Autodesk Inventor part; units mm, degrees
ref_plane "YZ Plane" through (0, 0, 0) normal (1, 0, 0) x (0, 1, 0)
ref_plane "XZ Plane" through (0, 0, 0) normal (0, 1, 0) x (-1, 0, 0)
ref_plane "XY Plane" through (0, 0, 0) normal (0, 0, 1) x (1, 0, 0)
sketch "Sketch1" plane through (0, 0, 0) normal (0, 0, 1) x (1, 0, 0)
  circle A0 centre (-0.2626, 0.8226) radius 5.775
  line L0 (-5.743, 8.5976) -> (11.2384, 8.5976)
  arc A1 (8.5691, -6.944) -> (11.2384, 8.5976) centre (11.2384, 0.5976) ccw
  line L1 (8.5691, -6.944) -> (-5.9413, -0.2275)
  line L2 (-5.743, 6.5976) -> (11.2384, 6.5976)
  arc A2 (9.3184, -5.0869) -> (11.2384, 6.5976) centre (11.2384, 0.5976) ccw
  line L3 (9.3184, -5.0869) -> (-5.9413, 1.9763)
  line L4 (-5.743, 8.5976) -> (-5.743, 6.5976)
  line L5 (-5.9413, 1.9763) -> (-5.9413, -0.2275)
  point P0 (0, 0)
  dimension "d6" = 11.55
  dimension "d0" = 6
  dimension "d2" = 2
  dimension "d3" = 90
extrude "Extrusion1" add sketch "Sketch1" along normal blind 10 contours L2 L4 L0 A1 L1 A0 L3 A2 | A0 L1 L5 L3 | A0 L5 L3
properties part number "01_Laser_Clamp_OnOffSwitch"
Could you check a few things on this model? Use its own coordinates, in mm. A direction names the side the tool comes from. Give positions to 0.01 mm unless a question says otherwise; leave off trailing zeros. Write each loop counter-clockwise with the first axis right and the second up, starting at its lowest first coordinate (ties: lowest second). Pieces come first, ordered by that corner, then holes. Notation, with made-up numbers: (76.25, 63.25) - (124.25, 63.25) arc R36 cw to (124.25, 100.25) - close; hole circle Ø3 at (3.25, -2). An arc over 180 degrees is marked (long way). Use CSV: the item, a comma, the result in double quotes. Start each with the question number.
Item 1: For faces 4 (the face through (6, -4, 10)), 5 (the face through (-5.743, 8, 5)), 6 (the face through (1.795, -1.605, 4.93)), 7 (the face through (1.415, -3.633, 4.93)), 8 (the face through (3, 6.598, 5)), which set-ups out of +Z, -Z, +X, -X, +Y, -Y let a thin tool reach every point of the face, with its end or its side?
Item 2: I'm going to push flat-ended pins straight in: pin 1 (1.5 mm diameter, centred on x = 0, y = 5, fed in from +Z); pin 2 (2 mm diameter, centred on y = 8, z = 5.5, fed in from -X); pin 3 (2 mm diameter, centred on y = 5.5, z = 1, fed in from +X). Where does each tip first touch, or does it pass through?
Item 3: I want a section at A-A, the plane x = 15. Please give me the cut outline in (y, z), then the cut area to 3 significant figures.
Item 4: I want a section at C-C, the plane z = 6.25. Please give me the cut outline in (x, y).
Item 5: If I drill on line 1 along Y through (x, z) = (5, 0.75); line 2 along Y through (x, z) = (0.5, 8.25); line 3 along X through (y, z) = (-4.75, 9.25), over which ranges is the centre line in solid material (lowest first)?
Item 6: If we mould it in two halves opening along X, with no side actions, what happens to faces 1 (the face through (3, 8.598, 5)), 2 (the face through (17.18, -0.23, 4.93)), 3 (the face through (-5.941, 1, 5))? For each: pulls with the +X half, pulls with the -X half, needs draft (parallel to the pull), parting line crosses it, or undercut.
Item 7: I want a section at D-D, the plane y = 5.75. Please give me the cut outline in (x, z), then the cut area to 3 significant figures.
Item 8: I want a section at B-B, the plane y = -0.5. Please give me the cut outline in (x, z).
Findings:
1,face 4,"+Z, +X, -X, +Y, -Y"
1,face 5,"+Z, -Z, -X, +Y"
1,face 6,"+Z, -Z"
1,face 7,"+Z, -Z, -X, -Y"
1,face 8,"+Z, -Z, -X"
2,pin 1,"passes through"
2,pin 2,"stops at x = -5.74"
2,pin 3,"stops at x = 18.22"
3,outline,"(-6.46, 0) - (-4.08, 0) - (-4.08, 10) - (-6.46, 10) - close; (5.27, 0) - (7.66, 0) - (7.66, 10) - (5.27, 10) - close"
3,area,"47.7 mm2"
4,outline,"(-5.94, -0.23) - (8.57, -6.94) arc R8 ccw (long way) to (11.24, 8.6) - (-5.74, 8.6) - (-5.74, 6.6) - (11.24, 6.6) arc R6 cw (long way) to (9.32, -5.09) - (-5.94, 1.98) - close"
5,line 1,"y = -5.29 to -3.09, 6.6 to 8.6"
5,line 2,"y = -3.21 to -1.01, 6.6 to 8.6"
5,line 3,"x = 3.83 to 8.59, 13.96 to 17.19"
6,face 1,"needs draft"
6,face 2,"undercut"
6,face 3,"pulls with the -X half"
7,outline,"(14.31, 0) - (17.36, 0) - (17.36, 10) - (14.31, 10) - close"
7,area,"30.5 mm2"
8,outline,"(-5.35, 0) - (-0.59, 0) - (-0.59, 10) - (-5.35, 10) - close; (17.14, 0) - (19.16, 0) - (19.16, 10) - (17.14, 10) - close"
